from build123d import *

# Parameters (mm, degrees)
F1_DEPTH = 15
F2_R     = 1.99999
F3_SIZE  = 3


# Not quite as in the source:
# - a fillet or chamfer is up to 0.001 mm smaller than in the source, because OpenCascade refuses the exact size


with BuildPart() as f1:
    # F0 (on Top) → F1 (new body)
    with BuildSketch(Plane.XY):
        Polygon((0, 16), (0, 2), (1.5, 2), (1.5, 0), (6.2, 0), (6.2, 3.55), (5.2, 3.55), (5.2, 1.75), (4, 1.75), (4, 16.25), (5.2, 16.25), (5.2, 14.45), (6.2, 14.45), (6.2, 18), (1.5, 18), (1.5, 16), align=None)
    extrude(amount=F1_DEPTH)

    # F2 (radius 2 in the source; OpenCascade refuses exactly that, so slightly less here)
    f2_edges = [f1.edges().sort_by_distance(p)[0] for p in [
        (1.5, 0, 7.5),
        (1.5, 18, 7.5),
    ]]
    fillet(f2_edges, radius=F2_R)

    # F3
    f3_edges = [f1.edges().sort_by_distance(p)[0] for p in [
        (0, 9, 0),
        (0, 9, 15),
    ]]
    chamfer(f3_edges, length=F3_SIZE)


solid = f1.part
Part model, mm, in its own coordinate system. A direction names the side the tool comes from. Coordinates: 2 decimals unless noted, no trailing zeros. Loops run counter-clockwise (first coordinate to the right, second up) from the corner with the lowest first, then second, coordinate; pieces in that order, holes last. Notation, with made-up numbers: M 83,-13 L 98,-13 A32 cw 98,21 Z; hole C 11.25,56.5 d1. An arc over 180 degrees is marked long. Use a Markdown table: item, result. Add a question column.
Q1. Cut at D-D (y = 10.5). Write the cut outline in (x, z).
Q2. Which spindle directions (+Z, -Z, +X, -X, +Y, -Y) get a long thin tool onto all of the face, cutting with end or side? Do faces 1 (the flat face through (5.2, 3, 7)), 2 (the flat face through (5, 0, 7)), 3 (the flat face through (6, 3.55, 7)), 4 (the flat face through (1, 16, 7)). Say none if no direction does.
Q3. Mould opens along Y. For faces 5 (the flat face through (5, 16.25, 7)), 6 (the flat face through (6.2, 16, 7)), 7 (the flat face through (4, 9, 7)), 8 (the flat face through (1, 2, 7)) say: +Y half, -Y half, draft (parallel to the pull), parting line (faces both ways), or undercut.
Q4. Cut at B-B (y = 15). Write the cut outline in (x, z).
Q5. Probe L1, parallel to X at y = 2.25, z = 7.75; L2, parallel to Y at x = 6, z = 3.75; L3, parallel to Y at x = 4.5, z = 8.5. List the from-to ranges inside material, lowest first.
Q6. Cut at A-A (x = 5.75). Write the cut outline in (y, z), and give its area (4 significant figures).
Q7. Pin check, flat tips, straight feed: P1, Ø0.5, axis at x = 1, z = 9.5, coming from the -Y side; P2, Ø1.7, axis at x = 0.5, z = 9, coming from the +Y side; P3, Ø1.5, axis at x = 2.5, z = 8.5, coming from the -Y side; P4, Ø4.5, axis at y = 12.5, z = 6.5, coming from the +X side. Stop position of each tip, or through.
Worked out:
| question | item | result |
|---|---|---|
| 1 | outline | M 0,3 L 3,0 L 4,0 L 4,15 L 3,15 L 0,12 Z |
| 2 | face 1 | +Z, -Z |
| 2 | face 2 | +Z, -Z, +X, -X, -Y |
| 2 | face 3 | +Z, -Z, +X |
| 2 | face 4 | +Z, -Z, -X, +Y |
| 3 | face 5 | undercut |
| 3 | face 6 | draft |
| 3 | face 7 | undercut |
| 3 | face 8 | -Y half |
| 4 | outline | M 0,3 L 3,0 L 4,0 L 4,15 L 3,15 L 0,12 Z; M 5.2,0 L 6.2,0 L 6.2,15 L 5.2,15 Z |
| 5 | L1 | x = 0 to 4, 5.2 to 6.2 |
| 5 | L2 | y = 0 to 3.55, 14.45 to 18 |
| 5 | L3 | y = 0 to 1.75, 16.25 to 18 |
| 6 | outline | M 0,0 L 3.55,0 L 3.55,15 L 0,15 Z; M 14.45,0 L 18,0 L 18,15 L 14.45,15 Z |
| 6 | area | 106.5 mm2 |
| 7 | P1 | stops at y = 2 |
| 7 | P2 | stops at y = 16 |
| 7 | P3 | stops at y = 0.02 |
| 7 | P4 | stops at x = 6.2 |
